Read the model definition and answer for the solid it produces. Units are mm, in the model's axes. A direction names the side the tool comes from. Coordinates: 2 decimals unless noted, no trailing zeros. Loops run counter-clockwise (first coordinate to the right, second up) from the corner with the lowest first, then second, coordinate; pieces in that order, holes last. Notation, with made-up numbers: (80, 57) - (91, 57) arc R12 cw to (91, 72) - close; hole circle Ø7 at (-30, 46). An arc over 180 degrees is marked (long way). Use one line per item in the form item = value.
from build123d import *

# Parameters (mm, degrees)
CROQUIS1_W                 = 23
CROQUIS1_H                 = 12
SALIENTE_EXTRUIR1_DEPTH    = 19.5
CROQUIS2_W                 = 32
CROQUIS2_H                 = 12
SALIENTE_EXTRUIR2_DEPTH    = 2.5
CROQUIS3_W                 = 23
CROQUIS3_H                 = 12
SALIENTE_EXTRUIR3_DEPTH    = 3.5
CORTAR_EXTRUIR1_DEPTH      = 4.5
CORTAR_EXTRUIR1_DEPTH_BACK = 23
SALIENTE_EXTRUIR4_DEPTH    = 3
CROQUIS6_R                 = 2.5
SALIENTE_EXTRUIR5_DEPTH    = 3.5


with BuildPart() as part:
    # Croquis1 → Saliente-Extruir1 (new body)
    with BuildSketch(Plane(origin=(0, 0, 0), x_dir=(1, 0, 0), z_dir=(0, 1, 0))):
        Rectangle(CROQUIS1_W, CROQUIS1_H)
    extrude(amount=SALIENTE_EXTRUIR1_DEPTH)

    # Croquis2 → Saliente-Extruir2 (add)
    with BuildSketch(Plane(origin=(0, 19.5, 0), x_dir=(1, 0, 0), z_dir=(0, 1, 0))):
        Rectangle(CROQUIS2_W, CROQUIS2_H)
    extrude(amount=SALIENTE_EXTRUIR2_DEPTH)

    # Croquis3 → Saliente-Extruir3 (add)
    with BuildSketch(Plane(origin=(0, 22, 0), x_dir=(1, 0, 0), z_dir=(0, 1, 0))):
        Rectangle(CROQUIS3_W, CROQUIS3_H)
    extrude(amount=SALIENTE_EXTRUIR3_DEPTH)

    # Croquis4 → Cortar-Extruir1 (cut, two sides)
    with BuildSketch(Plane(origin=(0, 22, 0), x_dir=(1, 0, 0), z_dir=(0, 1, 0))) as cortar_extruir1_sk:
        with BuildLine():
            Line((-16, 2.161008353), (-16, -2.161008353))
            ThreePointArc((-16, -2.161008353), (-12.243002427, 0), (-16, 2.161008353))
        make_face()
        with BuildLine():
            Line((16, 2.161008353), (16, -2.161008353))
            ThreePointArc((16, -2.161008353), (12.243002427, 0), (16, 2.161008353))
        make_face()
    extrude(amount=CORTAR_EXTRUIR1_DEPTH, mode=Mode.SUBTRACT)
    extrude(cortar_extruir1_sk.sketch, amount=-CORTAR_EXTRUIR1_DEPTH_BACK, mode=Mode.SUBTRACT)

    # Croquis5 → Saliente-Extruir4 (add)
    with BuildSketch(Plane(origin=(0, 25.5, 0), x_dir=(1, 0, 0), z_dir=(0, 1, 0))):
        with BuildLine():
            ThreePointArc((-1.805877758, 2.861817604), (-10.905877758, 0), (-1.805877758, -2.861817604))
            ThreePointArc((-1.805877758, -2.861817604), (2.094122242, 0), (-1.805877758, 2.861817604))
        make_face()
    extrude(amount=SALIENTE_EXTRUIR4_DEPTH)

    # Croquis6 → Saliente-Extruir5 (add)
    with BuildSketch(Plane(origin=(0, 28.5, 0), x_dir=(1, 0, 0), z_dir=(0, 1, 0))):
        with Locations((-5.905877758, 0)):
            Circle(CROQUIS6_R)
    extrude(amount=SALIENTE_EXTRUIR5_DEPTH)


solid = part.part
Item 1: The part is cut by section C-C on y = 3.5. Give the vertices of the cut face in (x, z), plus the area to 3 significant figures.
Results below:
outline = (-11.5, -6) - (11.5, -6) - (11.5, 6) - (-11.5, 6) - close
area = 276 mm²
Item 2: Each of these flat-tipped pins is pushed along its axis until it touches: P1, Ø5, axis at x = 13.5, z = 3, coming from the +Y side; P2, Ø1, axis at y = 24.5, z = 0.5, coming from the -X side; P3, Ø3.5, axis at x = 0.5, z = 2.5, coming from the +Y side; P4, Ø2, axis at x = -14, z = -1, coming from the -Y side. Where does it stop, or does it pass through?
Results below:
P1 = 25.5
P2 = -11.5
P3 = 28.5
P4 = through
Item 3: The part is cut by section A-A on z = 0. Give the vertices of the cut face in (x, y).
Results below:
outline = (-12.24, 19.5) - (-11.5, 19.5) - (-11.5, 0) - (11.5, 0) - (11.5, 19.5) - (12.24, 19.5) - (12.24, 22) - (11.5, 22) - (11.5, 25.5) - (2.09, 25.5) - (2.09, 28.5) - (-3.41, 28.5) - (-3.41, 32) - (-8.41, 32) - (-8.41, 28.5) - (-10.91, 28.5) - (-10.91, 25.5) - (-11.5, 25.5) - (-11.5, 22) - (-12.24, 22) - close
Item 4: Which of the six approach directions +Z, -Z, +X, -X, +Y, -Y give full straight-line access (tool end or side, diameter ignored) to faces 4 (the flat face through (-11.5, 10, 0)), 5 (the flat face through (-12, 22, 0)), 6 (the cylindrical face through (2.093, 26.979, 0.079)), 7 (the flat face through (11.5, 24, 0)), 8 (the flat face through (12, 19.5, 0))?
Results below:
face_4 = +Z, -Z, -X, -Y
face_5 = +Z, -Z, -X, +Y
face_6 = +Y
face_7 = +Z, -Z, +X, +Y
face_8 = +Z, -Z, +X, -Y
Item 5: The part is cut by section D-D on x = -7. Give the vertices of the cut face in (y, z).
Results below:
outline = (0, -6) - (25.5, -6) - (25.5, -4.88) - (28.5, -4.88) - (28.5, -2.25) - (32, -2.25) - (32, 2.25) - (28.5, 2.25) - (28.5, 4.88) - (25.5, 4.88) - (25.5, 6) - (0, 6) - close
Item 6: Find the intervals of material crossed by L1, parallel to Y at x = 0, z = -1; L2, parallel to X at y = 24, z = 3.75; L3, parallel to X at y = 21.55, z = 0, in increasing order.
Results below:
L1 = 0 to 28.5
L2 = -11.5 to 11.5
L3 = -12.24 to 12.24
Item 7: The part is cut by section B-B on x = -0.5. Give the vertices of the cut face in (y, z), plus the area to 3 significant figures.
Results below:
outline = (0, -6) - (25.5, -6) - (25.5, -2.97) - (28.5, -2.97) - (28.5, 2.97) - (25.5, 2.97) - (25.5, 6) - (0, 6) - close
area = 324 mm²
Item 8: For a pull along X with two mould halves and no side action, classify faces 1 (the flat face through (-6, 32, 0)), 2 (the flat face through (16, 21, -4)), 3 (the cylindrical face through (12.244, 20.768, 0.073)) as +X half, -X half, draft (parallel to the pull), parting line (faces both ways), or undercut.
Results below:
face_1 = draft
face_2 = +X half
face_3 = undercut
